Geometry: see drawing. Coordinates: mm, zero at the bounding-box minimum. A direction names the side the tool comes from. Round coordinates to 2 decimals unless told otherwise and drop trailing zeros. Loops run counter-clockwise (first coordinate to the right, second up) from the corner with the lowest first, then second, coordinate; pieces in that order, holes last. Notation, with made-up numbers: (30, 75) - (84, 75) arc R22 ccw to (84, 93) - close; hole circle Ø6 at (47.25, 32.25). An arc over 180 degrees is marked (long way). Return JSON: item names as keys, results as strings. Group by question number.
1. Section A-A on y = 30. Return loops of the section in (x, z), and give its area (4 significant figures).
2. Section D-D on x = 57. Return loops of the section in (y, z), and give its area (3 significant figures).
3. Material intervals for probe 1 along X at (y, z) = (30, 22); probe 2 along Y at (x, z) = (155, 29.5); probe 3 along X at (y, z) = (6, 36), sorted ascending.
4. Section C-C on x = 143. Return loops of the section in (y, z).
5. First-contact query: pin 1 Ø5 at (x, y) = (35, 39) entering from +Z; pin 2 Ø5 at (x, y) = (105, 49) entering from +Z; pin 3 Ø3 at (x, y) = (99, 10.5) entering from +Z. Flat tips, straight axial feed; report the tip coordinate or a pass-through.
6. Section B-B on z = 30. Return loops of the section in (x, y).
7. Set-up query: the marked faces 1, 2 and 3. Return all of +Z, -Z, +X, -X, +Y, -Y with unobstructed straight access to the full face (end or side cutting, diameter ignored); none if empty.
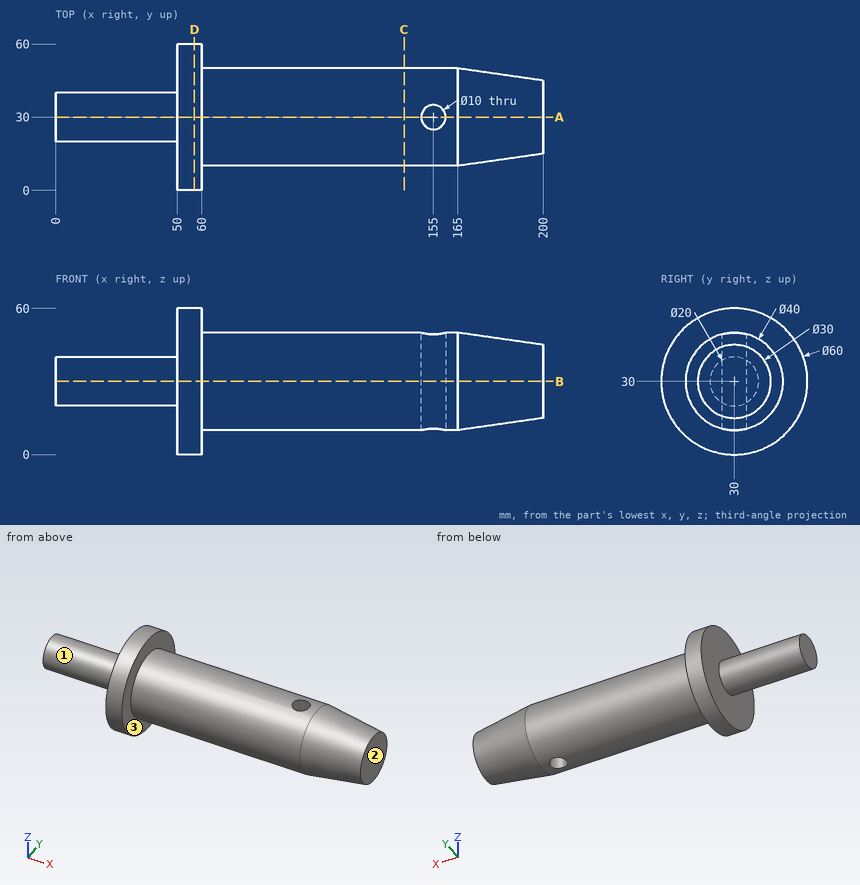
Taken from the geometry:
{
 "1": {"outline": "(0, 20) - (50, 20) - (50, 0) - (60, 0) - (60, 10) - (150, 10) - (150, 50) - (60, 50) - (60, 60) - (50, 60) - (50, 40) - (0, 40) - close; (160, 10) - (165, 10) - (200, 15) - (200, 45) - (165, 50) - (160, 50) - close", "area": "6,625 mm2"},
 "2": {"outline": "circle Ø60 at (30, 30)", "area": "2,830 mm2"},
 "3": {"probe 1": "0 to 150, 160 to 200", "probe 2": "10.01 to 25, 35 to 49.99", "probe 3": "50 to 60"},
 "4": {"outline": "circle Ø40 at (30, 30)"},
 "5": {"pin 1": "z = 37.6", "pin 2": "z = 41.3", "pin 3": "z = 38.72"},
 "6": {"outline": "(0, 20) - (50, 20) - (50, 0) - (60, 0) - (60, 10) - (165, 10) - (200, 15) - (200, 45) - (165, 50) - (60, 50) - (60, 60) - (50, 60) - (50, 40) - (0, 40) - close; hole circle Ø10 at (155, 30)"},
 "7": {"face 1": "-X", "face 2": "+Z, -Z, +X, +Y, -Y", "face 3": "+X"}
}
